```python
from build123d import *

# Parameters (mm, degrees)
SKETCH_1_R          = 1.75
SKETCH_1_R_2        = 1.55
EXTRUDE_1_DEPTH     = 7.6
SKETCH_2_R          = 0.5
CUT_EXTRUDE_1_DEPTH = 10
FILLET_1_R          = 5
EXTRUDE_START       = 27.7
SKETCH_4_R          = 1.55
EXTRUDE_2_DEPTH     = 27.7
SKETCH_6_R          = 2.5
CUT_EXTRUDE_2_DEPTH = 5
FILLET_START        = -29
FILLET_2_DEPTH      = 29
FILLET_2_2_DEPTH    = 9


with BuildPart() as part:
    # 草图1 → 凸台-拉伸1 (new body)
    with BuildSketch(Plane.XY):
        with BuildLine():
            Line((48.25, -17.561563803), (48.25, 0))
            ThreePointArc((48.25, 0), (45.781945765, 15.234038926), (38.630271835, 28.909593528))
            Line((38.630271835, 28.909593528), (28.062669438, 10.605969263))
            ThreePointArc((28.062669438, 10.605969263), (7.764571353, -28.977774789), (-29.605969263, -4.846295906))
            Line((-29.605969263, -4.846295906), (-46.660254038, 5))
            Line((-46.660254038, 5), (-60, 5))
            Line((-60, 5), (-60, -20.45))
            Line((-60, -20.45), (-48, -20.45))
            Line((-48, -20.45), (-48, -28.65))
            Line((-48, -28.65), (-52.5, -28.65))
            Line((-52.5, -28.65), (-52.5, -46.25))
            Line((-52.5, -46.25), (24.177543768, -46.25))
            Line((24.177543768, -46.25), (48.25, -17.561563803))
        make_face()
        with Locations(Location((-31.466251763, -31.466251763, 0), (0, 0, 180))):
            Circle(SKETCH_1_R, mode=Mode.SUBTRACT)
        with Locations(Location((-55, -15.45, 0), (0, 0, 180))):
            Circle(SKETCH_1_R_2, mode=Mode.SUBTRACT)
        with Locations(Location((0, -42.5, 0), (0, 0, 180))):
            Circle(SKETCH_1_R, mode=Mode.SUBTRACT)
        with Locations(Location((31.466251763, -31.466251763, 0), (0, 0, 180))):
            Circle(SKETCH_1_R, mode=Mode.SUBTRACT)
        with Locations(Location((-55, -0.45, 0), (0, 0, 180))):
            Circle(SKETCH_1_R_2, mode=Mode.SUBTRACT)
        with Locations(Location((-44.5, 0, 0), (0, 0, 180))):
            Circle(SKETCH_1_R, mode=Mode.SUBTRACT)
        with Locations(Location((44.5, 0, 0), (0, 0, 180))):
            Circle(SKETCH_1_R, mode=Mode.SUBTRACT)
    extrude(amount=EXTRUDE_1_DEPTH)

    # 草图2 → 切除-拉伸1 (cut)
    with BuildSketch(Plane(origin=(0, 0, 0), x_dir=(-1, 0, 0), z_dir=(0, 0, -1))):
        with Locations((48, -20.45)):
            Circle(SKETCH_2_R)
        with Locations((48, -28.65)):
            Circle(SKETCH_2_R)
    extrude(amount=-CUT_EXTRUDE_1_DEPTH, mode=Mode.SUBTRACT)

    # 圆角1
    fillet_1_edges = [part.edges().sort_by_distance(p)[0] for p in [
        (48.25, -17.561563803, 3.8),
        (-46.660254038, 5, 3.8),
        (-29.605969263, -4.846295906, 3.8),
        (28.062669438, 10.605969263, 3.8),
        (38.630271835, 28.909593528, 3.8),
    ]]
    fillet(fillet_1_edges, radius=FILLET_1_R)

    # 草图4 → 凸台-拉伸2 (add)
    with BuildSketch(Plane(origin=(0, 0, 0), x_dir=(-1, 0, 0), z_dir=(0, 0, -1)).offset(EXTRUDE_START)):
        with BuildLine():
            Line((60, 5), (48.241579576, 5))
            ThreePointArc((48.241579576, 5), (48.490086253, -0.980579006), (48, -6.946221995))
            Line((48, -6.946221995), (48, -20.45))
            Line((48, -20.45), (60, -20.45))
            Line((60, -20.45), (60, 5))
        make_face()
        with Locations((55, -15.45)):
            Circle(SKETCH_4_R, mode=Mode.SUBTRACT)
        with Locations((55, -0.45)):
            Circle(SKETCH_4_R, mode=Mode.SUBTRACT)
    extrude(amount=-EXTRUDE_2_DEPTH)

    # 草图6 → 切除-拉伸2 (cut)
    with BuildSketch(Plane.XZ.offset(20.45)):
        with Locations(Location((-55, -21.35, 0), (0, 0, 270))):
            Circle(SKETCH_6_R)
        with Locations(Location((-55, -6.35, 0), (0, 0, 270))):
            Circle(SKETCH_6_R)
    extrude(amount=-CUT_EXTRUDE_2_DEPTH, mode=Mode.SUBTRACT)

    # 圆角2: read off the stored shape, not the designer's step
    # 圆角2 outline → 圆角2 (cut)
    with BuildSketch(Plane.XY.offset(FILLET_START)):
        with BuildLine():
            Line((-49, -20.45), (-48, -20.45))
            Line((-48, -20.45), (-48, -19.45))
            ThreePointArc((-48, -19.45), (-48.292893219, -20.157106781), (-49, -20.45))
        make_face()
        with BuildLine():
            Line((-60, -20.45), (-59, -20.45))
            ThreePointArc((-59, -20.45), (-59.707106781, -20.157106781), (-60, -19.45))
            Line((-60, -19.45), (-60, -20.45))
        make_face()
        with BuildLine():
            Line((-60, 5), (-60, 4))
            ThreePointArc((-60, 4), (-59.707106781, 4.707106781), (-59, 5))
            Line((-59, 5), (-60, 5))
        make_face()
        with BuildLine():
            ThreePointArc((-49.338119137, 5), (-48.602997351, 4.67793507), (-48.341389458, 3.919191919))
            ThreePointArc((-48.341389458, 3.919191919), (-48.294508108, 4.45987518), (-48.241579576, 5))
            Line((-48.241579576, 5), (-49.338119137, 5))
        make_face()
    extrude(amount=FILLET_2_DEPTH, mode=Mode.SUBTRACT)

    # Fillet 2 2 outline → Fillet 2 2 (cut)
    with BuildSketch(Plane.XY):
        with BuildLine():
            ThreePointArc((-48.477859457, -20.302859457), (-48.728761597, -20.412512196), (-49, -20.45))
            Line((-49, -20.45), (-48.5, -20.45))
            ThreePointArc((-48.5, -20.45), (-48.494433883, -20.375601507), (-48.477859457, -20.302859457))
        make_face()
        with BuildLine():
            Line((-60, -20.45), (-59, -20.45))
            ThreePointArc((-59, -20.45), (-59.707106781, -20.157106781), (-60, -19.45))
            Line((-60, -19.45), (-60, -20.45))
        make_face()
        with BuildLine():
            Line((-60, 5), (-60, 4))
            ThreePointArc((-60, 4), (-59.707106781, 4.707106781), (-59, 5))
            Line((-59, 5), (-60, 5))
        make_face()
        with BuildLine():
            Line((-52.5, -28.65), (-52.5, -29.65))
            ThreePointArc((-52.5, -29.65), (-52.207106781, -28.942893219), (-51.5, -28.65))
            Line((-51.5, -28.65), (-52.5, -28.65))
        make_face()
        with BuildLine():
            Line((-52.5, -46.25), (-51.5, -46.25))
            ThreePointArc((-51.5, -46.25), (-52.207106781, -45.957106781), (-52.5, -45.25))
            Line((-52.5, -45.25), (-52.5, -46.25))
        make_face()
        with BuildLine():
            ThreePointArc((24.477280553, -45.89278761), (24.133854372, -46.156307787), (23.71123611, -46.25))
            Line((23.71123611, -46.25), (24.177543768, -46.25))
            Line((24.177543768, -46.25), (24.477280553, -45.89278761))
        make_face()
    extrude(amount=FILLET_2_2_DEPTH, mode=Mode.SUBTRACT)


solid = part.part
```
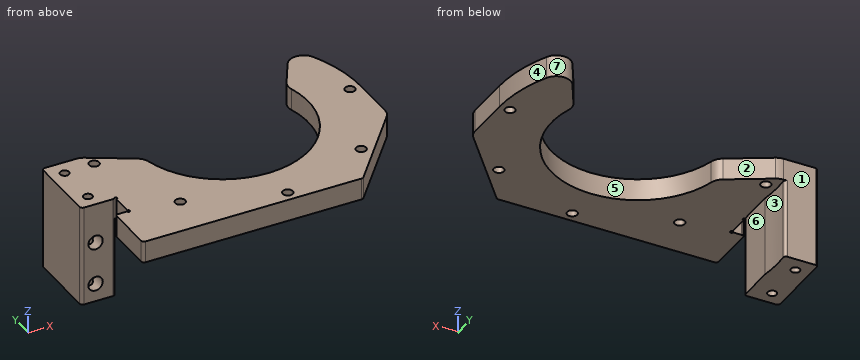
Geometry: final body of the model. Coordinates: model frame, mm. Face numbers are marked on the shaded views. A direction names the side the tool comes from. Round coordinates to 2 decimals unless told otherwise and drop trailing zeros. Write each loop counter-clockwise with the first axis right and the second up, starting at its lowest first coordinate (ties: lowest second). Pieces come first, ordered by that corner, then holes. Notation, with made-up numbers: M 63.25,-29.75 L 67.25,-29.75 A9 cw 67.25,-16.75 Z; hole C 57,46 d6. An arc over 180 degrees is marked long. Answer in a Markdown table with one row per item. Add a question column.
(1) Ray query, L1, parallel to Y at x = -55, z = 2; L2, parallel to Z at x = -55, y = -18.1; L3, parallel to X at y = -16.7, z = -21.35. Return the intervals inside material, ascending.
(2) Cut plane A-A, the plane y = -25.5. Return the cut outline in (x, z).
(3) Contact query for flat-ended pins moving along their axis: pin 1 (4 mm diameter, centred on x = -55, y = -15.45, fed in from +Z); pin 2 (6.5 mm diameter, centred on x = -55, z = -21.35, fed in from -Y); pin 3 (10 mm diameter, centred on y = -14.5, z = -13, fed in from +X); pin 4 (0.9 mm diameter, centred on x = -50, z = 3.5, fed in from +Y). Output: stop coordinate, or through.
(4) Cut plane B-B, the plane z = -17.5. Return the cut outline in (x, y).
(5) Draft query along X for the marked faces 5, 6 and 7. Return one class per face: pulls with the +X half, pulls with the -X half, needs draft (parallel to the pull), parting line crosses it, or undercut.
(6) Cut plane D-D, the plane x = 7. Return the cut outline in (y, z).
(7) Cut plane C-C, the plane z = -6.35. Return the cut outline in (x, y), then the cut area to 3 significant figures.
(8) Reachability of the marked faces 1, 2, 3 and 4 from +Z, -Z, +X, -X, +Y, -Y: full face, straight path, thin tool, end or side. Return the list, or none.
Established:
| question | item | result |
|---|---|---|
| 1 | L1 | -20.45 to -17, -13.9 to -2, 1.1 to 5 |
| 1 | L2 | -27.7 to -23.85, -18.85 to -8.85, -3.85 to 7.6 |
| 1 | L3 | -60 to -57.5, -52.5 to -48 |
| 2 | outline | M -48,0 L -15.8,0 L -15.8,7.6 L -48,7.6 Z; M 15.8,0 L 41.59,0 L 41.59,7.6 L 15.8,7.6 Z |
| 3 | pin 1 | z = 7.6 |
| 3 | pin 2 | y = -20.45 |
| 3 | pin 3 | x = -48 |
| 3 | pin 4 | y = 5 |
| 4 | outline | M -60,-19.45 A1 ccw -59,-20.45 L -49,-20.45 A1 ccw -48,-19.45 L -48,-6.95 A48.5 cw -48.34,3.92 A1 ccw -49.34,5 L -59,5 A1 ccw -60,4 Z; hole C -55,-15.45 d3.1; hole C -55,-0.45 d3.1 |
| 5 | face 5 | undercut |
| 5 | face 6 | pulls with the +X half |
| 5 | face 7 | parting line crosses it |
| 6 | outline | M -46.25,0 L -29.17,0 L -29.17,7.6 L -46.25,7.6 Z |
| 7 | outline | M -60,-19.45 A1 ccw -59,-20.45 L -57.5,-20.45 L -57.5,-15.45 L -56.55,-15.45 A1.55 cw -53.45,-15.45 L -52.5,-15.45 L -52.5,-20.45 L -49,-20.45 A1 ccw -48,-19.45 L -48,-6.95 A48.5 cw -48.34,3.92 A1 ccw -49.34,5 L -59,5 A1 ccw -60,4 Z; hole C -55,-0.45 d3.1 |
| 7 | area | 264 mm² |
| 8 | face 1 | +Z, -Z, -X, +Y |
| 8 | face 2 | +Z, -Z, +Y |
| 8 | face 3 | -Z, +X |
| 8 | face 4 | +Z, -Z, +X, +Y |
